```python
from build123d import *

# Parameters (mm, degrees)
F0_W     = 152.4
F0_H     = 101.6
F1_DEPTH = 12.7
F2_W     = 146.05
F2_H     = 6.35
F3_DEPTH = 6.35
F5_DEPTH = 6.35


with BuildPart() as f1:
    # F0 (on Front) → F1 (new body)
    with BuildSketch(Plane.XZ):
        Rectangle(F0_W, F0_H)
    extrude(amount=F1_DEPTH)

    # F2 (on face) → F3 (cut)
    with BuildSketch(Plane(origin=(0, 0, 0), x_dir=(-1, 0, 0), z_dir=(0, 1, 0))):
        with Locations((0, -41.275)):
            Rectangle(F2_W, F2_H)
    extrude(amount=-F3_DEPTH, mode=Mode.SUBTRACT)

    # F4 (on face) → F5 (cut)
    with BuildSketch(Plane(origin=(0, 0, 0), x_dir=(-1, 0, 0), z_dir=(0, 1, 0))):
        with BuildLine():
            Line((76.2, 19.05), (76.2, 31.75))
            ThreePointArc((76.2, 31.75), (69.85, 25.4), (76.2, 19.05))
        make_face()
        with BuildLine():
            Line((76.2, -6.35), (76.2, 6.35))
            ThreePointArc((76.2, 6.35), (69.85, 0), (76.2, -6.35))
        make_face()
        with BuildLine():
            ThreePointArc((76.2, -19.05), (69.85, -25.4), (76.2, -31.75))
            Line((76.2, -31.75), (76.2, -19.05))
        make_face()
        with BuildLine():
            ThreePointArc((-76.2, -31.75), (-69.85, -25.4), (-76.2, -19.05))
            Line((-76.2, -19.05), (-76.2, -31.75))
        make_face()
        with BuildLine():
            ThreePointArc((-76.2, -6.35), (-69.85, 0), (-76.2, 6.35))
            Line((-76.2, 6.35), (-76.2, -6.35))
        make_face()
        with BuildLine():
            Line((-76.2, 31.75), (-76.2, 19.05))
            ThreePointArc((-76.2, 19.05), (-69.85, 25.4), (-76.2, 31.75))
        make_face()
    extrude(amount=-F5_DEPTH, mode=Mode.SUBTRACT)


solid = f1.part
```
Geometry check sheet. Reference: the model listing, model coordinates, mm. A direction names the side the tool comes from. Coordinates: 2 decimals unless noted, no trailing zeros. Order: outer loops, then holes, each group sorted by start corner. A loop starts at its lowest first (then second) coordinate and runs counter-clockwise, first axis right, second up. Notation, with made-up numbers: (-22.75, 20.25) - (24.25, 20.25) arc R22 ccw to (24.25, 29.25) - close; hole circle Ø6 at (64, 73). An arc over 180 degrees is marked (long way). Use one line per item in the form item = value.
1. Draft check along Z on faces 6 (the face through (1, -3, -38.1)), 7 (the face through (-1, -6, -50.8)), 8 (the face through (-1, 0, 1)). Enter one of: pulls with the +Z half, pulls with the -Z half, needs draft (parallel to the pull), parting line crosses it, or undercut.
Here are the results:
face_6 = undercut
face_7 = pulls with the -Z half
face_8 = needs draft
2. Section check B-B (z = 0). Record the boundary of the cut face in (x, y).
Here are the results:
outline = (-76.2, -12.7) - (76.2, -12.7) - (76.2, -6.35) - (69.85, -6.35) - (69.85, 0) - (-69.85, 0) - (-69.85, -6.35) - (-76.2, -6.35) - close
3. Gauge pin test, flat end, axial feed: pin 1 (5 mm diameter, centred on x = 74.5, z = 25.5, fed in from +Y). Record the tip position at first contact, or that the pin passes through.
Here are the results:
pin_1 = -6.35
4. Access from +Z, -Z, +X, -X, +Y, -Y to the whole of each face (thin tool, end or side, straight path). Record for faces 1 (the face through (-74, -6.35, 0)), 2 (the face through (76.2, -8, -1)), 3 (the face through (74, -6.35, 25)), 4 (the face through (-1, -12.7, 1)), 5 (the face through (1, -3, -44.45)).
Here are the results:
face_1 = -X, +Y
face_2 = +Z, -Z, +X, +Y, -Y
face_3 = +X, +Y
face_4 = +Z, -Z, +X, -X, -Y
face_5 = +Y
5. Section check A-A (x = -41). Record the boundary of the cut face in (y, z).
Here are the results:
outline = (-12.7, -50.8) - (0, -50.8) - (0, -44.45) - (-6.35, -44.45) - (-6.35, -38.1) - (0, -38.1) - (0, 50.8) - (-12.7, 50.8) - close
6. Scan lines: line 1 (Z direction, x = 62, y = -5.5); line 2 (X direction, y = -1.5, z = -41) (3 decimals); line 3 (Y direction, x = 30.5, z = -43.5). Record each from-to range of solid material in increasing order.
Here are the results:
line_1 = -50.8 to -44.45, -38.1 to 50.8
line_2 = -76.2 to -73.025, 73.025 to 76.2
line_3 = -12.7 to -6.35
